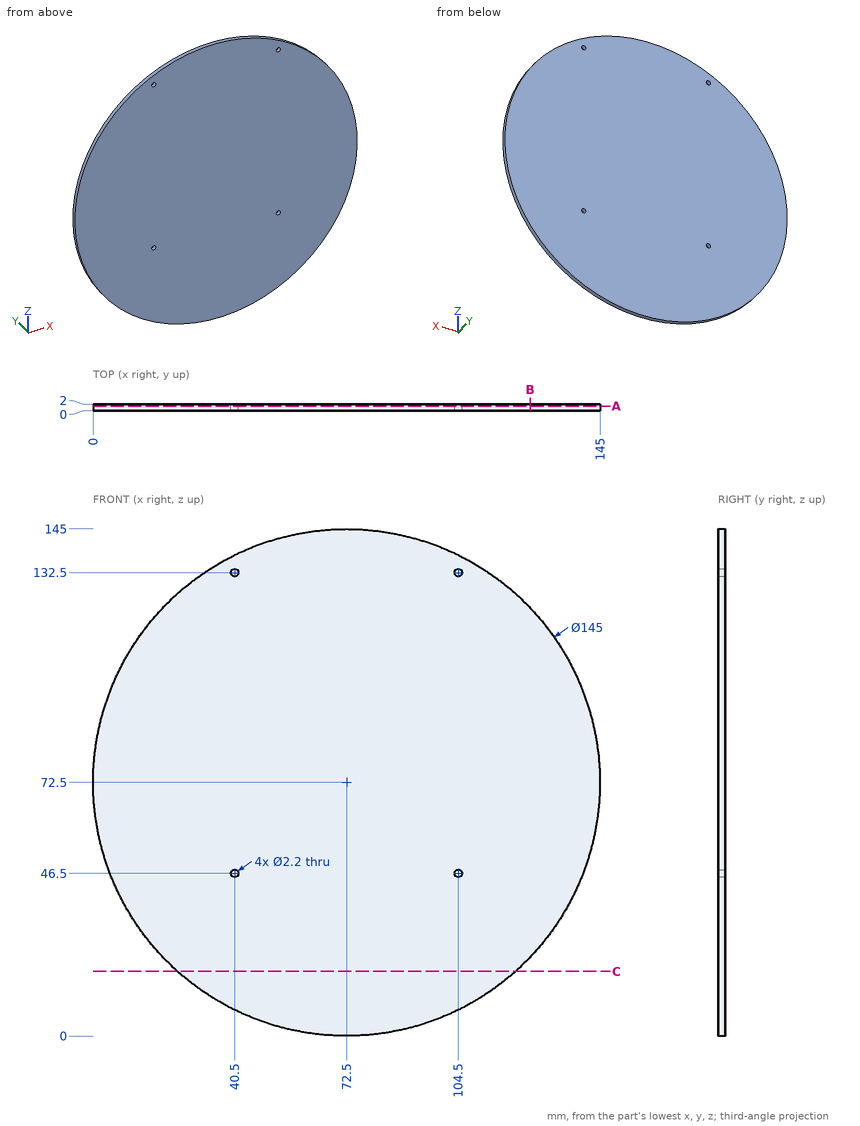
Answer from the drawing. Dimensions are ordinates in mm from the lowest x, y and z of the part. Round coordinates to 2 decimals unless told otherwise and drop trailing zeros. Loops run counter-clockwise (first coordinate to the right, second up) from the corner with the lowest first, then second, coordinate; pieces in that order, holes last. Notation, with made-up numbers: (59, 60.5) - (96, 60.5) arc R14 ccw to (96, 86.5) - close; hole circle Ø7 at (-5, 65). An arc over 180 degrees is marked (long way). Return JSON: item names as keys, results as strings. Group by question number.
1. The part is cut by section B-B on x = 125. Determine the outline of the cut face in (y, z).
2. The part is cut by section A-A on y = 1.4. Determine the outline of the cut face in (x, z).
3. Consider probe 1 along X at (y, z) = (0.5, 132.5); probe 2 along X at (y, z) = (0.6, 46.5); probe 3 along Z at (x, y) = (40.5, 1.3). Determine where each line is inside the solid, lowest interval first.
4. The part is cut by section C-C on z = 18.5. Determine the outline of the cut face in (x, y), then the cut area to 3 significant figures.
Resolved:
{
 "1": {"outline": "(0, 22.5) - (2, 22.5) - (2, 122.5) - (0, 122.5) - close"},
 "2": {"outline": "circle Ø145 at (72.5, 72.5); hole circle Ø2.2 at (40.5, 46.5); hole circle Ø2.2 at (40.5, 132.5); hole circle Ø2.2 at (104.5, 46.5); hole circle Ø2.2 at (104.5, 132.5)"},
 "3": {"probe 1": "x = 31.8 to 39.4, 41.6 to 103.4, 105.6 to 113.2", "probe 2": "x = 4.82 to 39.4, 41.6 to 103.4, 105.6 to 140.18", "probe 3": "z = 7.44 to 45.4, 47.6 to 131.4, 133.6 to 137.56"},
 "4": {"outline": "(24.12, 0) - (120.88, 0) - (120.88, 2) - (24.12, 2) - close", "area": "194 mm²"}
}
